Work out the finished part from the listing and answer in its coordinate system (mm). A direction names the side the tool comes from. Give positions to 0.01 mm unless a question says otherwise; leave off trailing zeros. Loops run counter-clockwise (first coordinate to the right, second up) from the corner with the lowest first, then second, coordinate; pieces in that order, holes last. Notation, with made-up numbers: (44, 28.25) - (65, 28.25) arc R28 cw to (65, 65.25) - close; hole circle Ø2 at (43, 41.25). An arc over 180 degrees is marked (long way). Use CSV: the item, a comma, the result in double quotes.
from build123d import *

# Parameters (mm, degrees)
CROQUIS1_W              = 40
CROQUIS1_H              = 45
SALIENTE_EXTRUIR1_DEPTH = 4.5
CROQUIS2_W              = 10
CROQUIS2_H              = 45
SALIENTE_EXTRUIR2_DEPTH = 5.5
REDONDEO1_R             = 1


with BuildPart() as part:
    # Croquis1 → Saliente-Extruir1 (new body)
    with BuildSketch(Plane.XY):
        Rectangle(CROQUIS1_W, CROQUIS1_H)
    extrude(amount=SALIENTE_EXTRUIR1_DEPTH)

    # Croquis2 → Saliente-Extruir2 (add)
    with BuildSketch(Plane(origin=(0, 0, 0), x_dir=(-1, 0, 0), z_dir=(0, 0, -1))):
        with Locations((-15, 0)):
            Rectangle(CROQUIS2_W, CROQUIS2_H)
        with Locations((15, 0)):
            Rectangle(CROQUIS2_W, CROQUIS2_H)
    extrude(amount=SALIENTE_EXTRUIR2_DEPTH)

    # Redondeo1
    redondeo1_edges = [part.edges().sort_by_distance(p)[0] for p in [
        (-20, 0, 4.5),
        (0, -22.5, 4.5),
        (20, 0, 4.5),
        (0, 22.5, 4.5),
    ]]
    fillet(redondeo1_edges, radius=REDONDEO1_R)


solid = part.part
Item 1: Given P1, Ø3, axis at x = -1.5, y = 15.5, coming from the -Z side, flat-ended and moving along its own axis, determine where the tip first touches the part or whether it passes through.
Determined:
P1,"stops at z = 0"
Item 2: Find the intervals of material crossed by line 1 (X direction, y = 11.5, z = -2); line 2 (Z direction, x = -6, y = -12); line 3 (X direction, y = -10, z = 4), in increasing order.
Determined:
line 1,"x = -20 to -10, 10 to 20"
line 2,"z = 0 to 4.5"
line 3,"x = -19.87 to 19.87"
Item 3: A cutting plane is placed at B-B on x = -7. Determine the outline of the cut face in (y, z).
Determined:
outline,"(-22.5, 0) - (22.5, 0) - (22.5, 3.5) arc R1 ccw to (21.5, 4.5) - (-21.5, 4.5) arc R1 ccw to (-22.5, 3.5) - close"
Item 4: A cutting plane is placed at C-C on y = 11.5. Determine the outline of the cut face in (x, z), and give its area (3 significant figures).
Determined:
outline,"(-20, -5.5) - (-10, -5.5) - (-10, 0) - (10, 0) - (10, -5.5) - (20, -5.5) - (20, 3.5) arc R1 ccw to (19, 4.5) - (-19, 4.5) arc R1 ccw to (-20, 3.5) - close"
area,"290 mm²"
Item 5: The mould has two halves that part along X. Classify faces 1 (the cylindrical face through (-19.715, 0.315, 4.199)), 2 (the flat face through (0, 0, 0)), 3 (the flat face through (15, 0, -5.5)): pulls with the +X half, pulls with the -X half, needs draft (parallel to the pull), parting line crosses it, or undercut.
Determined:
face 1,"pulls with the -X half"
face 2,"undercut"
face 3,"needs draft"
Item 6: A cutting plane is placed at A-A on z = -1.75. Determine the outline of the cut face in (x, y).
Determined:
outline,"(-20, -22.5) - (-10, -22.5) - (-10, 22.5) - (-20, 22.5) - close; (10, -22.5) - (20, -22.5) - (20, 22.5) - (10, 22.5) - close"
Item 7: For faces 4 (the flat face through (-20, 0, -1)), 5 (the flat face through (-10, 0, -3)), determine the directions among +Z, -Z, +X, -X, +Y, -Y from which every point of the face is accessible in a straight line to the end or side of a thin tool.
Determined:
face 4,"+Z, -Z, -X, +Y, -Y"
face 5,"-Z, +Y, -Y"
